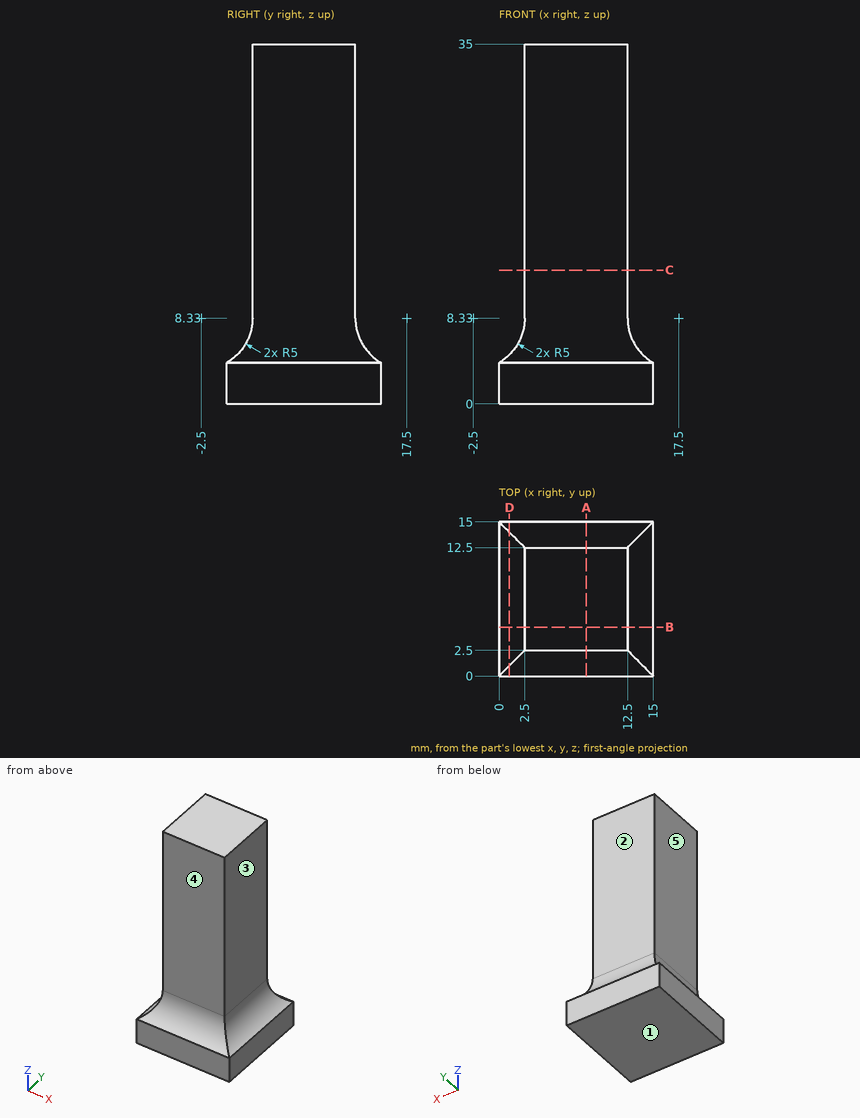
Check sheet for the drawn part. Datum: minimum x, y, z corner. Units: mm. A direction names the side the tool comes from. Give positions to 0.01 mm unless a question says otherwise; leave off trailing zeros. Order: outer loops, then holes, each group sorted by start corner. A loop starts at its lowest first (then second) coordinate and runs counter-clockwise, first axis right, second up. Notation, with made-up numbers: (-39.75, 62) - (-18.75, 62) arc R18 ccw to (-18.75, 66) - close; hole circle Ø7 at (-9, -24.5). An arc over 180 degrees is marked (long way). Answer in a Markdown table with one row per item. Add a question column.
Q1. Cross-section at A-A, the plane x = 8.5. Enter the section's corners in (y, z), then the cut area to 3 significant figures.
Q2. Cross-section at C-C, the plane z = 13. Enter the section's corners in (x, y), then the cut area to 3 significant figures.
Q3. Cross-section at D-D, the plane x = 1. Enter the section's corners in (y, z), then the cut area to 3 significant figures.
Q4. Material ranges on probe 1 along Y at (x, z) = (12.25, 29.5); probe 2 along X at (y, z) = (2.25, 6), recorded low to high. Write a range as from..to.
Q5. Tool access check on the marked faces 1, 2, 3, 4 and 5. Record the directions out of +Z, -Z, +X, -X, +Y, -Y that give a thin tool (end or side, any length) a straight path to the whole face; none if there is none.
Q6. Gauge pin test, flat ends, axial feed: pin 1 (1.5 mm diameter, centred on y = 7.5, z = 22.5, fed in from -X); pin 2 (5 mm diameter, centred on x = 9, z = 17.5, fed in from -Y); pin 3 (5 mm diameter, centred on x = 7, z = 27, fed in from +Y). Record the tip position at first contact, or that the pin passes through.
Check values:
| question | item | result |
|---|---|---|
| 1 | outline | (0, 0) - (15, 0) - (15, 4) arc R5 cw to (12.5, 8.33) - (12.5, 35) - (2.5, 35) - (2.5, 8.33) arc R5 cw to (0, 4) - close |
| 1 | area | 376 mm^2 |
| 2 | outline | (2.5, 2.5) - (12.5, 2.5) - (12.5, 12.5) - (2.5, 12.5) - close |
| 2 | area | 100 mm^2 |
| 3 | outline | (0, 0) - (15, 0) - (15, 4) arc R5 cw to (14, 4.76) - (1, 4.76) arc R5 cw to (0, 4) - close |
| 3 | area | 70.6 mm^2 |
| 4 | probe 1 | y = 2.5..12.5 |
| 4 | probe 2 | x = 1.92..13.08 |
| 5 | face 1 | -Z, +X, -X, +Y, -Y |
| 5 | face 2 | +Z, +X, -X, +Y |
| 5 | face 3 | +Z, +X, +Y, -Y |
| 5 | face 4 | +Z, +X, -X, -Y |
| 5 | face 5 | +Z, -X, +Y, -Y |
| 6 | pin 1 | stops at x = 2.5 |
| 6 | pin 2 | stops at y = 2.5 |
| 6 | pin 3 | stops at y = 12.5 |
